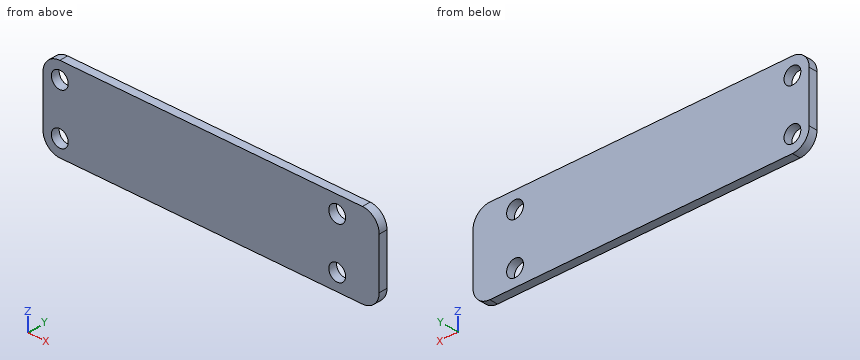
Autodesk Fusion 360 part; units mm, degrees
sketch "Sketch1" plane through (0, 0, 0) normal (0, 1, 0) x (1, 0, 0)
  line L0 (100, 25) -> (-100, 25)
  line L1 (-100, 25) -> (-100, -25)
  line L2 (-100, -25) -> (100, -25)
  line L3 (100, -25) -> (100, 25)
  line L4 (100, 25) -> (-100, -25) construction
  line L5 (-100, 25) -> (100, -25) construction
  dimension "d1" = 200
  dimension "d2" = 50
extrude "Extrude1" add sketch "Sketch1" along normal blind 5
fillet "Fillet1" radius 10 4 edges at (-100, 2.5, 25) (-100, 2.5, -25) (100, 2.5, -25) (100, 2.5, 25)
sketch "Sketch2" plane through (0, 5, 0) normal (0, 1, 0) x (-1, 0, 0)
  arc A0 (-90, 25) -> (-100, 15) centre (-90, 15) ccw
  line L0 (-100, 15) -> (-100, -15)
  arc A1 (-100, -15) -> (-90, -25) centre (-90, -15) ccw
  line L1 (-90, -25) -> (90, -25)
  arc A2 (90, -25) -> (100, -15) centre (90, -15) ccw
  line L2 (100, -15) -> (100, 15)
  arc A3 (100, 15) -> (90, 25) centre (90, 15) ccw
  line L3 (90, 25) -> (-90, 25)
  circle A4 centre (90, -15) radius 5
  circle A5 centre (90, 15) radius 5
  circle A6 centre (-75, -15) radius 5
  circle A7 centre (-75, 15) radius 5
  dimension "d6" = 10
  dimension "d7" = 15
extrude "Extrude2" cut sketch "Sketch2" against normal through all contours A4 | A5 | A6 | A7
Could you check a few things on this model? Use its own coordinates, in mm. Give positions to 0.01 mm unless a question says otherwise; leave off trailing zeros. Write each loop counter-clockwise with the first axis right and the second up, starting at its lowest first coordinate (ties: lowest second). Pieces come first, ordered by that corner, then holes. Notation, with made-up numbers: (87, 8.25) -> (100, 8.25) arc R24 cw to (100, 34.25) -> close; hole circle Ø2 at (0, 17.25). An arc over 180 degrees is marked (long way). Answer as a JSON object with one key per item and string values.
Q1. Please list where these lines run through material, in increasing order: L1, parallel to Z at x = 75, y = 3.95; L2, parallel to X at y = 1, z = 11; L3, parallel to X at y = 1.2, z = 12.
Taken from the geometry:
{"L1": "z = -25 to -20, -10 to 10, 20 to 25", "L2": "x = -100 to -93, -87 to 72, 78 to 100", "L3": "x = -100 to -94, -86 to 71, 79 to 100"}
Q2. Will these pins go through, and if not, where does the flat tip stop? pin 1 Ø1 at (y, z) = (2, -18.5) entering from +X; pin 2 Ø6 at (x, z) = (75, -15) entering from -Y.
Taken from the geometry:
{"pin 1": "stops at x = 99.54", "pin 2": "passes through"}
Q3. Suppose I cut it at A-A on x = 75. Write out the boundary of the cut face in (y, z), then the cut area to 3 significant figures.
Taken from the geometry:
{"outline": "(0, -25) -> (5, -25) -> (5, -20) -> (0, -20) -> close; (0, -10) -> (5, -10) -> (5, 10) -> (0, 10) -> close; (0, 20) -> (5, 20) -> (5, 25) -> (0, 25) -> close", "area": "150 mm²"}
Q4. Suppose I cut it at B-B on y = 2.2. Write out the boundary of the cut face in (x, z).
Taken from the geometry:
{"outline": "(-100, -15) arc R10 ccw to (-90, -25) -> (90, -25) arc R10 ccw to (100, -15) -> (100, 15) arc R10 ccw to (90, 25) -> (-90, 25) arc R10 ccw to (-100, 15) -> close; hole circle Ø10 at (-90, -15); hole circle Ø10 at (-90, 15); hole circle Ø10 at (75, -15); hole circle Ø10 at (75, 15)"}
